Can you work these out from the model? Positions are in its coordinate system, mm. A direction names the side the tool comes from. Round coordinates to 2 decimals unless told otherwise and drop trailing zeros. Order: outer loops, then holes, each group sorted by start corner. A loop starts at its lowest first (then second) coordinate and runs counter-clockwise, first axis right, second up.
from build123d import *

# Parameters (mm, degrees)
ESQUISSE1_W             = 25
ESQUISSE1_H             = 40
BOSS_EXTRU_2_DEPTH      = 15
ESQUISSE3_W             = 19
ESQUISSE3_H             = 35
ENL_V_MAT_EXTRU_4_DEPTH = 16
ESQUISSE4_R             = 1
BOSS_EXTRU_3_DEPTH      = 10
ESQUISSE5_R             = 4
ENL_V_MAT_EXTRU_5_DEPTH = 26


with BuildPart() as part:
    # Esquisse1 → Boss.-Extru.2 (new body)
    with BuildSketch(Plane.XY):
        with Locations((12.5, -20)):
            Rectangle(ESQUISSE1_W, ESQUISSE1_H)
    extrude(amount=BOSS_EXTRU_2_DEPTH)

    # Esquisse3 → Enlèv. mat.-Extru.4 (cut, through all)
    with BuildSketch(Plane.XY):
        with Locations((12.5, -17.5)):
            Rectangle(ESQUISSE3_W, ESQUISSE3_H)
    extrude(amount=ENL_V_MAT_EXTRU_4_DEPTH, mode=Mode.SUBTRACT)

    # Esquisse4 → Boss.-Extru.3 (add)
    with BuildSketch(Plane(origin=(0, -35, 0), x_dir=(1, 0, 0), z_dir=(0, 1, 0))):
        with Locations((7.5, -7.5)):
            Circle(ESQUISSE4_R)
    extrude(amount=BOSS_EXTRU_3_DEPTH)

    # Esquisse5 → Enlèv. mat.-Extru.5 (cut, through all)
    with BuildSketch(Plane.ZY):
        with Locations((7.5, -18)):
            Circle(ESQUISSE5_R)
    extrude(amount=-ENL_V_MAT_EXTRU_5_DEPTH, mode=Mode.SUBTRACT)


solid = part.part
(1) If we mould it in two halves opening along Z, with no side actions, what happens to faces 1 (the face through (23, -26, 15)), 2 (the face through (1.479, -14.034, 6.979)), 3 (the face through (22, -14, 6)), 4 (the face through (7.37, -30.07, 6.51))? For each: pulls with the +Z half, pulls with the -Z half, needs draft (parallel to the pull), parting line crosses it, or undercut.
(2) I'm going to push flat-ended pins straight in: pin 1 Ø2 at (x, y) = (9, -29.5) entering from -Z; pin 2 Ø4.5 at (y, z) = (-25, 5) entering from -X; pin 3 Ø0.6 at (x, z) = (8, 8) entering from +Y. Where does each tip first touch, or does it pass through?
(3) I want a section at D-D, the plane y = -18. List the corners of the cut face in (x, z) for me, plus the area to 3 significant figures.
(4) I want a section at A-A, the plane z = 7.5. List the corners of the cut face in (x, y) for me.
(5) I want a section at C-C, the plane y = -8. List the corners of the cut face in (x, z) for me.
(6) On a 3-axis mill with a long thin cutter (end or side, diameter ignored), from which of +Z, -Z, +X, -X, +Y, -Y can I reach the whole of each face in a straight line? I mean faces 5 (the face through (1, 0, 7)), 6 (the face through (7, -25, 7)). Say none if no direction works.
(7) Please list where these lines run through material, in increasing order: probe 1 along Y at (x, z) = (2.3, 7.5); probe 2 along X at (y, z) = (-20, 11.5); probe 3 along Y at (x, z) = (14.5, 3.75).
(8) I want a section at B-B, the plane y = -33. List the corners of the cut face in (x, z) for me, plus the area to 3 significant figures.
Ans:
1. face 1: pulls with the +Z half
1. face 2: undercut
1. face 3: needs draft
1. face 4: parting line crosses it
2. pin 1: stops at z = 6.63
2. pin 2: stops at x = 0
2. pin 3: stops at y = -25
3. outline: (0, 0) - (3, 0) - (3, 3.5) - (0, 3.5) - close; (0, 11.5) - (3, 11.5) - (3, 15) - (0, 15) - close; (22, 0) - (25, 0) - (25, 3.5) - (22, 3.5) - close; (22, 11.5) - (25, 11.5) - (25, 15) - (22, 15) - close
3. area: 42.0 mm2
4. outline: (0, -40) - (25, -40) - (25, -22) - (22, -22) - (22, -35) - (8.5, -35) - (8.5, -25) - (6.5, -25) - (6.5, -35) - (3, -35) - (3, -22) - (0, -22) - close; (0, -14) - (3, -14) - (3, 0) - (0, 0) - close; (22, -14) - (25, -14) - (25, 0) - (22, 0) - close
5. outline: (0, 0) - (3, 0) - (3, 15) - (0, 15) - close; (22, 0) - (25, 0) - (25, 15) - (22, 15) - close
6. face 5: +Z, -Z, +X, -X, +Y
6. face 6: +Z, -Z, +Y
7. probe 1: y = -40 to -22, -14 to 0
7. probe 2: x = 0 to 3, 22 to 25
7. probe 3: y = -40 to -35
8. outline: (0, 0) - (3, 0) - (3, 15) - (0, 15) - close; circle Ø2 at (7.5, 7.5); (22, 0) - (25, 0) - (25, 15) - (22, 15) - close
8. area: 93.1 mm2
